from build123d import *

# Parameters (mm, degrees)
SKETCH_2_W             = 64.02174429
SKETCH_2_H             = 9.248919907
CUT_EXTRUDE_1_DEPTH    = 49
HOLE_WIZARD_M4_2_D     = 3.3
HOLE_WIZARD_M4_2_DEPTH = 5.5
HOLE_WIZARD_M4_2_TIP   = 0.991420021
HOLE_WIZARD_M6_2_D     = 5
HOLE_WIZARD_M6_2_DEPTH = 5.5
HOLE_WIZARD_M6_2_TIP   = 1.502151548


with BuildPart() as part:
    # 草图1 → 旋转1 (revolve)
    with BuildSketch(Plane(origin=(0, 0, 0), x_dir=(1, 0, 0), z_dir=(0, 1, 0)), mode=Mode.PRIVATE) as revolve_1_sk:
        Polygon((32.5, 7.5), (32.5, -7.5), (23.5, -7.5), (23.5, -3), (24.1, -3), (24.1, -2), (19, -2), (19, 2), (24.1, 2), (24.1, 3), (23.5, 3), (23.5, 7.5), align=None)
    revolve(revolve_1_sk.sketch.rotate(Axis((0, 0, -31.9390681), (0, 0, 1)), 180), axis=Axis((0, 0, -31.9390681), (0, 0, 1)))  # turned: the seam where the file's is

    # 草图2 → 切除-拉伸1 (cut)
    with BuildSketch(Plane.XY.offset(7.5)):
        with Locations((-1.141100508, 36.374459954)):
            Rectangle(SKETCH_2_W, SKETCH_2_H)
        with Locations((-1.141100508, -36.374459954)):
            Rectangle(SKETCH_2_W, SKETCH_2_H)
    extrude(amount=-CUT_EXTRUDE_1_DEPTH, mode=Mode.SUBTRACT)

    # M4 螺纹孔2
    with Locations(Plane(origin=(0, 31.75, 0), x_dir=(1, 0, 0), z_dir=(0, 1, 0))):
        with Locations((0, 0)):
            Hole(HOLE_WIZARD_M4_2_D / 2, depth=HOLE_WIZARD_M4_2_DEPTH)
            with Locations((0, 0, -(HOLE_WIZARD_M4_2_DEPTH + HOLE_WIZARD_M4_2_TIP / 2))):  # 118° drill point
                Cone(0, HOLE_WIZARD_M4_2_D / 2, HOLE_WIZARD_M4_2_TIP, mode=Mode.SUBTRACT)

    # M6 螺纹孔2
    with Locations(Plane(origin=(0, -31.75, 0), x_dir=(-1, 0, 0), z_dir=(0, -1, 0))):
        with Locations((0, 0)):
            Hole(HOLE_WIZARD_M6_2_D / 2, depth=HOLE_WIZARD_M6_2_DEPTH)
            with Locations((0, 0, -(HOLE_WIZARD_M6_2_DEPTH + HOLE_WIZARD_M6_2_TIP / 2))):  # 118° drill point
                Cone(0, HOLE_WIZARD_M6_2_D / 2, HOLE_WIZARD_M6_2_TIP, mode=Mode.SUBTRACT)


solid = part.part
Design review of the part built by this model. Coordinates are the model's own, in mm. A direction names the side the tool comes from. Give positions to 0.01 mm unless a question says otherwise; leave off trailing zeros. Write each loop counter-clockwise with the first axis right and the second up, starting at its lowest first coordinate (ties: lowest second). Pieces come first, ordered by that corner, then holes. Notation, with made-up numbers: M -0.5,36.5 L 42.5,36.5 A21 ccw 42.5,50.5 Z; hole C 30.25,-32 d4. An arc over 180 degrees is marked long. Answer as a JSON object with one key per item and string values. Group by question number.
1) Clearance check with flat-ended pins moving along their axes: pin 1 Ø8 at (y, z) = (-8, -2) entering from -X; pin 2 Ø3 at (x, z) = (0, 0) entering from +Y; pin 3 Ø1 at (y, z) = (-18.5, -0.5) entering from +X; pin 4 Ø5 at (x, z) = (-1.5, 1.5) entering from -Y. State where each tip first meets the part, or that it passes through.
2) Mouldability with a two-part tool opening along Z and no side actions: class faces 4 (the face through (-14, 21, 7.5)), 5 (the face through (5.2, 23.1, 3)), 6 (the face through (3.06, -23.3, -5.28)) as released by +Z, released by -Z, zero draft, split by the parting line, or undercut.
3) Tool access review of faces 1 (the face through (1.216, 28.962, -1.115)), 2 (the face through (-0.54, -28.96, 2.44)), 3 (the face through (17.76, -16.29, -2.51)): name each direction out of +Z, -Z, +X, -X, +Y, -Y from which nothing blocks a thin tool from reaching the whole face with its end or side.
4) We need section C-C (x = 3.5). Give the boundary of the cut face in (y, z), and give its area (3 significant figures).
5) We need section A-A (y = 0). Give the boundary of the cut face in (x, z), and give its area (3 significant figures).
6) We need section D-D (x = 26). Give the boundary of the cut face in (y, z).
7) We need section B-B (z = 6.5). Give the boundary of the cut face in (x, y), and give its area (3 significant figures).
8) For line 1 along Z through (x, y) = (0, -28.1); line 2 along Y through (x, z) = (0, 2.7); line 3 along Y through (x, z) = (0, -4.25), list the stretches that pass through material, from the lowest coordinate up.
Answer key:
{
 "1": {"pin 1": "stops at x = -32.25", "pin 2": "stops at y = 26.16", "pin 3": "stops at x = 27.06", "pin 4": "stops at y = -31.75"},
 "2": {"face 4": "released by +Z", "face 5": "undercut", "face 6": "zero draft"},
 "3": {"face 1": "+Y", "face 2": "-Y", "face 3": "none"},
 "4": {"outline": "M -31.75,-7.5 L -23.24,-7.5 L -23.24,-3 L -23.84,-3 L -23.84,-2 L -18.67,-2 L -18.67,2 L -23.84,2 L -23.84,3 L -23.24,3 L -23.24,7.5 L -31.75,7.5 Z; M 18.67,-2 L 23.84,-2 L 23.84,-3 L 23.24,-3 L 23.24,-7.5 L 31.75,-7.5 L 31.75,7.5 L 23.24,7.5 L 23.24,3 L 23.84,3 L 23.84,2 L 18.67,2 Z", "area": "289 mm²"},
 "5": {"outline": "M -32.5,-7.5 L -23.5,-7.5 L -23.5,-3 L -24.1,-3 L -24.1,-2 L -19,-2 L -19,2 L -24.1,2 L -24.1,3 L -23.5,3 L -23.5,7.5 L -32.5,7.5 Z; M 19,-2 L 24.1,-2 L 24.1,-3 L 23.5,-3 L 23.5,-7.5 L 32.5,-7.5 L 32.5,7.5 L 23.5,7.5 L 23.5,3 L 24.1,3 L 24.1,2 L 19,2 Z", "area": "304 mm²"},
 "6": {"outline": "M -19.5,-7.5 L 19.5,-7.5 L 19.5,7.5 L -19.5,7.5 Z"},
 "7": {"outline": "M -6.94,-31.75 L 6.94,-31.75 A32.5 ccw 6.94,31.75 L -6.94,31.75 A32.5 ccw Z; hole C 0,0 d47", "area": "1,570 mm²"},
 "8": {"line 1": "z = -7.5 to -2.5, 2.5 to 7.5", "line 2": "y = -31.75 to -24.1, 24.1 to 31.75", "line 3": "y = -31.75 to -23.5, 23.5 to 31.75"}
}
